The model under review builds one solid part; all positions refer to its coordinate system, in mm. Face numbers are marked on the shaded views. A direction names the side the tool comes from. Give positions to 0.01 mm unless a question says otherwise; leave off trailing zeros. Order: outer loops, then holes, each group sorted by start corner. A loop starts at its lowest first (then second) coordinate and runs counter-clockwise, first axis right, second up. Notation, with made-up numbers: (39, 42) - (84, 42) arc R25 cw to (84, 59) - close; hole circle Ø5 at (-18.75, 31.5). An arc over 180 degrees is marked (long way). Put each result on its own line as item: value.
```python
from build123d import *

# Parameters (mm, degrees)
THICKEN1_T1        = 12
CUT_EXTRUDE1_DEPTH = 727.760405867
CIRPATTERN1_COUNT  = 6
CIRPATTERN2_COUNT  = 8


with BuildPart() as body_1:
    # Surface-Revolve1: a surface, the sketch's curves turned about an axis
    with BuildLine(Plane.XY, mode=Mode.PRIVATE) as surface_revolve1_1_path:
        Line((79.5, 0), (172.5, 0))
        ThreePointArc((172.5, 0), (213.5312381, -30.75), (254.5624762, 0))
        Line((254.5624762, 0), (299.5624762, 0))
        ThreePointArc((299.5624762, 0), (331.357632054, 9.117114231), (353.490118977, 33.697731193))
        Line((353.490118977, 33.697731193), (410.214525599, 150))
        Line((410.214525599, 150), (497.75, 150))
    surface_revolve1_1 = Shell.revolve(surface_revolve1_1_path.wire(), 360, Axis((0, 0, 0), (0, 1, 0)))
    add(Solid.thicken(surface_revolve1_1, THICKEN1_T1))

    # Sketch2 → Cut-Extrude1 (cut, through all)
    with BuildSketch(Plane.XZ.offset(-138)):
        with BuildLine():
            ThreePointArc((-416.77522058, 272.12768696), (-208.753886972, 361.809245054), (-27, 497.017165197))
            ThreePointArc((-27, 497.017165197), (-248.752750649, 431.13470232), (-416.77522058, 272.12768696))
        make_face()
        with BuildLine():
            ThreePointArc((0, 480), (-15, 465), (0, 450))
            Line((0, 450), (0, 480))
        make_face()
        with BuildLine():
            Line((0, 480), (0, 450))
            ThreePointArc((0, 450), (10.606601718, 454.393398282), (15, 465))
            ThreePointArc((15, 465), (10.606601718, 475.606601718), (0, 480))
        make_face()
    cut_extrude1 = extrude(amount=-CUT_EXTRUDE1_DEPTH, mode=Mode.SUBTRACT)

    # CirPattern1: Cut-Extrude1 ×6 about axis
    cirpattern1_axis = Axis((0, 0, 0), (0, 1, 0))
    for i in range(1, CIRPATTERN1_COUNT):
        add(cut_extrude1.rotate(cirpattern1_axis, i * 360 / CIRPATTERN1_COUNT), mode=Mode.SUBTRACT)

    # Sketch5 → Ø25.0mm Dowel Hole1 (revolve, cut)
    with BuildSketch(Plane(origin=(0, -12, 121.5), x_dir=(0, 0, -1), z_dir=(1, 0, 0))):
        Polygon((0, 0), (0, 52.510757738), (12.5, 45), (12.5, 0), align=None)
    f_25_0mm_dowel_hole1 = revolve(axis=Axis((0, -18.35, 121.5), (0, 1, 0)), mode=Mode.SUBTRACT)

    # CirPattern2: Ø25.0mm Dowel Hole1 ×8 about axis
    cirpattern2_axis = Axis((0, 0, 0), (0, 1, 0))
    for i in range(1, CIRPATTERN2_COUNT):
        add(f_25_0mm_dowel_hole1.rotate(cirpattern2_axis, i * 360 / CIRPATTERN2_COUNT), mode=Mode.SUBTRACT)


solid = body_1.part
```
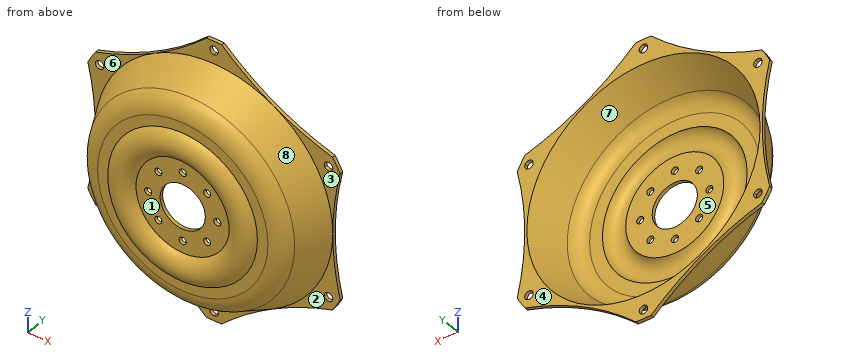
(1) Wall thickness on L1, parallel to Y at x = -7, z = -278; L2, parallel to Z at x = -178.5, y = 15; L3, parallel to Z at x = -126.5, y = 94: over which ranges is each line inside the solid? List them lowest first.
The answers:
L1: -12 to 0
L2: -307.75 to -288.49, 288.49 to 307.75
L3: -375.52 to -361.4, 361.4 to 375.52
(2) Take a section at A-A, the plane y = 75.5. Write out the cut boundary in (x, z), then the cut area to 3 significant figures.
The answers:
outline: circle Ø774.46 at (0, 0); hole circle Ø747.76 at (0, 0)
area: 31,900 mm^2
(3) The part is to be moulded in two halves that separate along Z. For the marked faces 6, 7 and 8, say which applies: pulls with the +Z half, pulls with the -Z half, needs draft (parallel to the pull), parting line crosses it, or undercut.
The answers:
face 6: needs draft
face 7: undercut
face 8: parting line crosses it
(4) For the marked faces 1, 2, 3, 4 and 5, list the 3-axis set-ups (+Z, -Z, +X, -X, +Y, -Y) from which the entire face can be reached by the end or side of a thin tool; tool diameter is ignored.
The answers:
face 1: -Y
face 2: -Z, +X, -Y
face 3: +Z, +X, -Y
face 4: +Z, -Z, +X, -X, +Y
face 5: +Y
(5) Clearance check with flat-ended pins moving along their axes: pin 1 Ø20 at (x, z) = (85.91, -85.91) entering from -Y; pin 2 Ø5 at (x, z) = (-131, -333.5) entering from -Y; pin 3 Ø3 at (x, y) = (288, 99) entering from -Z; pin 4 Ø5 at (x, z) = (42, 85.5) entering from +Y. State where each tip first meets the part, or that it passes through.
The answers:
pin 1: through
pin 2: y = 15.05
pin 3: z = -277.58
pin 4: y = 0
